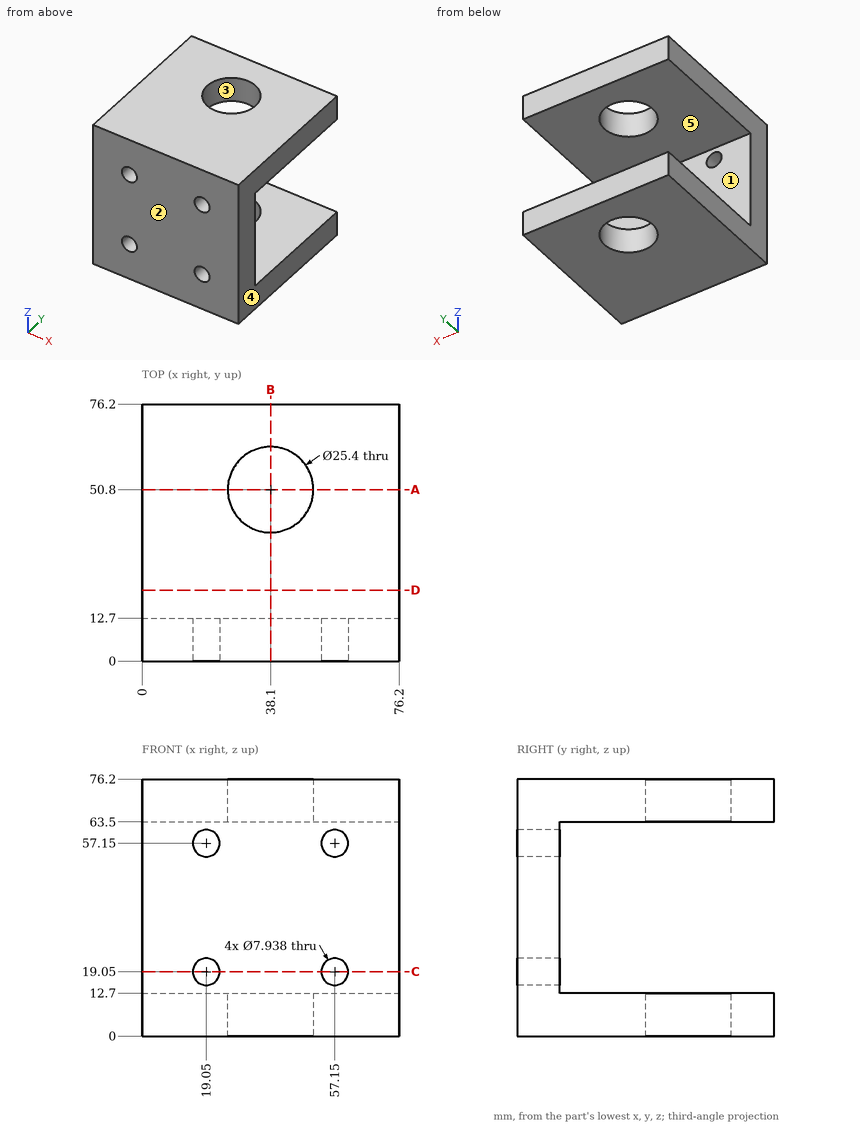
Part print with two shaded views. Sizes in mm from the minimum x, y, z corner. A direction names the side the tool comes from. Coordinates: 2 decimals unless noted, no trailing zeros. Order: outer loops, then holes, each group sorted by start corner. A loop starts at its lowest first (then second) coordinate and runs counter-clockwise, first axis right, second up.
(1) Drill centre lines: L1, parallel to X at y = 8, z = 57 (1 decimal); L2, parallel to Z at x = 19.05, y = 7.75; L3, parallel to Z at x = 20, y = 55. Where is each one in solid material? Low to high.
Solution:
L1: x = 0 to 15.1, 23 to 53.2, 61.1 to 76.2
L2: z = 0 to 15.08, 23.02 to 53.18, 61.12 to 76.2
L3: z = 0 to 12.7, 63.5 to 76.2
(2) Saw through at B-B, the plane x = 38.1. Write the cut outline in (y, z), and give its area (3 significant figures).
Solution:
outline: (0, 0) - (38.1, 0) - (38.1, 12.7) - (12.7, 12.7) - (12.7, 63.5) - (38.1, 63.5) - (38.1, 76.2) - (0, 76.2) - close; (63.5, 0) - (76.2, 0) - (76.2, 12.7) - (63.5, 12.7) - close; (63.5, 63.5) - (76.2, 63.5) - (76.2, 76.2) - (63.5, 76.2) - close
area: 1,940 mm2
(3) Mould opens along X. For the marked faces 3, 4 and 5 say: released by +X, released by -X, zero draft, split by the parting line, or undercut.
Solution:
face 3: undercut
face 4: released by +X
face 5: zero draft
(4) Saw through at C-C, the plane z = 19.05. Write the cut outline in (x, y).
Solution:
outline: (0, 0) - (15.08, 0) - (15.08, 12.7) - (0, 12.7) - close; (23.02, 0) - (53.18, 0) - (53.18, 12.7) - (23.02, 12.7) - close; (61.12, 0) - (76.2, 0) - (76.2, 12.7) - (61.12, 12.7) - close
(5) Pin check, flat tip, straight feed: pin 1 Ø20.5 at (x, y) = (38.1, 50.8) entering from -Z. Stop position of the tip, or through.
Solution:
pin 1: passes through
(6) Saw through at D-D, the plane y = 21. Write the cut outline in (x, z).
Solution:
outline: (0, 0) - (76.2, 0) - (76.2, 12.7) - (0, 12.7) - close; (0, 63.5) - (76.2, 63.5) - (76.2, 76.2) - (0, 76.2) - close
(7) Which spindle directions (+Z, -Z, +X, -X, +Y, -Y) get a long thin tool onto all of the face, cutting with end or side? Do the marked faces 1 and 2. Say none if no direction does.
Solution:
face 1: +X, -X, +Y
face 2: +Z, -Z, +X, -X, -Y
(8) Saw through at A-A, the plane y = 50.8. Write the cut outline in (x, z), and give its area (3 significant figures).
Solution:
outline: (0, 0) - (25.4, 0) - (25.4, 12.7) - (0, 12.7) - close; (0, 63.5) - (25.4, 63.5) - (25.4, 76.2) - (0, 76.2) - close; (50.8, 0) - (76.2, 0) - (76.2, 12.7) - (50.8, 12.7) - close; (50.8, 63.5) - (76.2, 63.5) - (76.2, 76.2) - (50.8, 76.2) - close
area: 1,290 mm2
